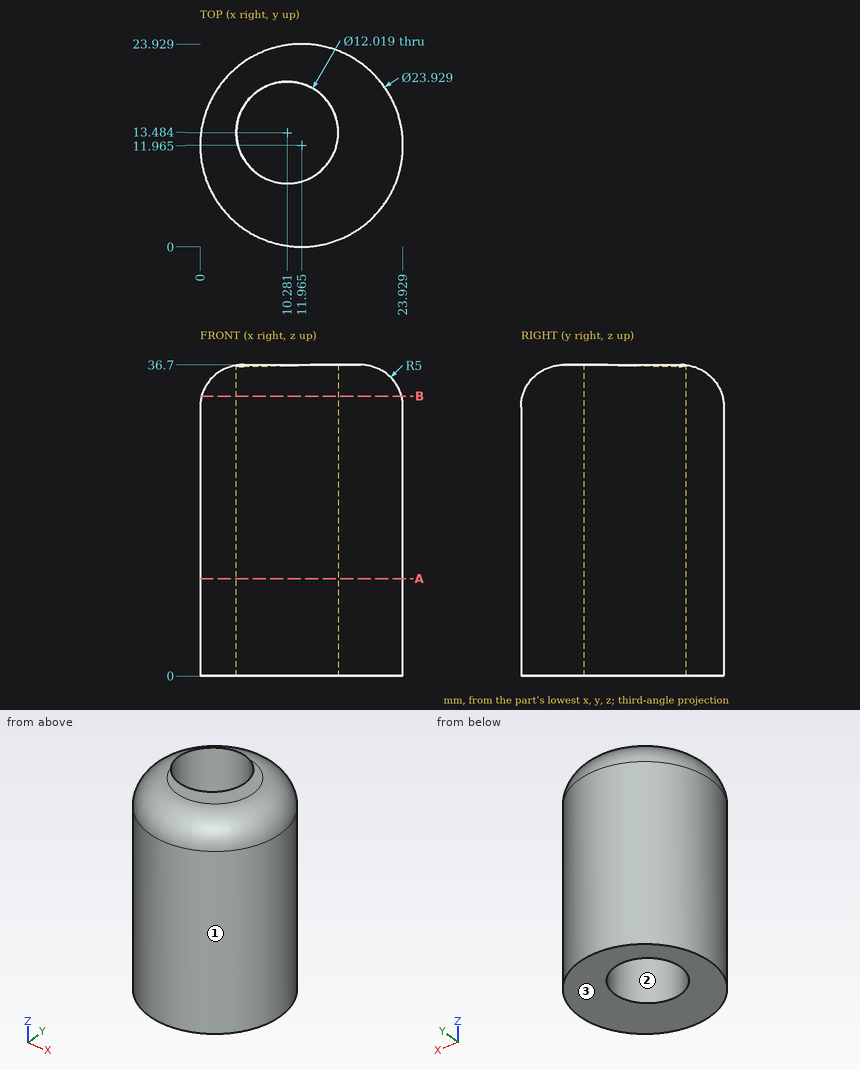
For this review, use the dimensioned drawing (mm, ordinates from the lowest corner) and the shaded views. Give positions to 0.01 mm unless a question says otherwise; leave off trailing zeros. Write each loop counter-clockwise with the first axis right and the second up, starting at its lowest first coordinate (ties: lowest second). Pieces come first, ordered by that corner, then holes. Notation, with made-up numbers: M 65.25,87.5 L 109.25,87.5 A28 ccw 109.25,125.5 Z; hole C -21.5,79 d10. An arc over 180 degrees is marked long. Answer as a JSON object with one key per item and string values. Group by question number.
1) We need section B-B (z = 33). Give the boundary of the cut face in (x, y) (1 decimal).
2) Mouldability with a two-part tool opening along X and no side actions: class the marked faces 1, 2 and 3 as released by +X, released by -X, zero draft, split by the parting line, or undercut.
3) For line 1 along Y through (x, z) = (7.25, 6.5) (1 decimal); line 2 along X through (y, z) = (9.75, 12.5) (1 decimal); line 3 along X through (y, z) = (12.25, 30) (1 decimal), list the stretches that pass through material, from the lowest coordinate up.
4) We need section A-A (z = 11.5). Give the boundary of the cut face in (x, y) (1 decimal).
5) Clearance check with flat-ended pins moving along their axes: pin 1 Ø1 at (x, z) = (3, 18.5) entering from +Y; pin 2 Ø1.5 at (x, z) = (17.5, 23.5) entering from +Y; pin 3 Ø1 at (x, y) = (18, 3.5) entering from +Z; pin 4 Ø5 at (x, y) = (8.5, 10.5) entering from -Z. State where each tip first meets the part, or that it passes through.
Answer key:
{
 "1": {"outline": "C 12,12 d23.6; hole C 10.3,13.5 d12"},
 "2": {"face 1": "split by the parting line", "face 2": "undercut", "face 3": "zero draft"},
 "3": {"line 1": "y = 1 to 8.3, 18.7 to 23", "line 2": "x = 0.2 to 5.6, 15 to 23.7", "line 3": "x = 0 to 4.4, 16.2 to 23.9"},
 "4": {"outline": "C 12,12 d23.9; hole C 10.3,13.5 d12"},
 "5": {"pin 1": "stops at y = 20.42", "pin 2": "stops at y = 22.93", "pin 3": "stops at z = 35.75", "pin 4": "passes through"}
}
